```python
from build123d import *

# Parameters (mm, degrees)
SKETCH1_R           = 8.75
BOSS_EXTRUDE1_DEPTH = 13
CUT_EXTRUDE1_REACH  = 19.948
SKETCH2_R           = 2.5
SKETCH3_R           = 4.05
CUT_EXTRUDE2_DEPTH  = 3
CHAMFER1_SIZE       = 0.5


with BuildPart() as part:
    # Sketch1 → Boss-Extrude1 (new body)
    with BuildSketch(Plane(origin=(0, 0, 0), x_dir=(1, 0, 0), z_dir=(0, 1, 0))):
        with Locations(Location((0, 0, 0), (0, 0, 90))):
            Circle(SKETCH1_R)
    extrude(amount=BOSS_EXTRUDE1_DEPTH)

    # Sketch2 → Cut-Extrude1 (cut, up to next)
    with BuildSketch(Plane(origin=(0, 13, 0), x_dir=(1, 0, 0), z_dir=(0, 1, 0)), mode=Mode.PRIVATE) as cut_extrude1_sk1:
        with Locations(Location((0, 0, 0), (0, 0, 270))):
            Circle(SKETCH2_R)
    cut_extrude1_tool1 = extrude(cut_extrude1_sk1.sketch, amount=-CUT_EXTRUDE1_REACH, mode=Mode.PRIVATE) & part.part
    add(cut_extrude1_tool1.solids().sort_by_distance((0, 13, 0))[0], mode=Mode.SUBTRACT)

    # Sketch3 → Cut-Extrude2 (cut)
    with BuildSketch(Plane(origin=(0, 13, 0), x_dir=(1, 0, 0), z_dir=(0, 1, 0))):
        with Locations(Location((0, 0, 0), (0, 0, 270))):
            Circle(SKETCH3_R)
    cut_extrude2 = extrude(amount=-CUT_EXTRUDE2_DEPTH, mode=Mode.SUBTRACT)

    # Mirror3: Cut-Extrude2 across plane
    add(cut_extrude2.mirror(Plane.ZX.offset(6.5)), mode=Mode.SUBTRACT)

    # Chamfer1
    chamfer1_edges = [part.edges().sort_by_distance(p)[0] for p in [
        (0, 13, -4.05),
        (0, 0, -4.05),
    ]]
    chamfer(chamfer1_edges, length=CHAMFER1_SIZE)


solid = part.part
```
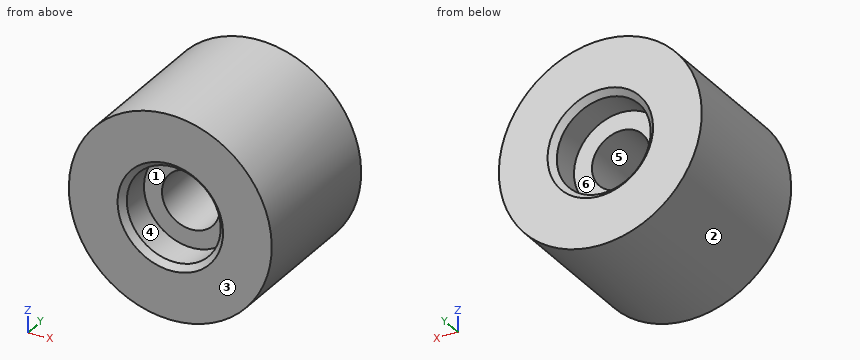
Check sheet for the modelled part. Datum: model origin and axes. Units: mm. Face numbers are marked on the shaded views. A direction names the side the tool comes from. Give positions to 0.01 mm unless a question says otherwise; leave off trailing zeros. Write each loop counter-clockwise with the first axis right and the second up, starting at its lowest first coordinate (ties: lowest second). Pieces come first, ordered by that corner, then holes.
Item 1: Cross-section at D-D (y = 8.5). Enter the section's corners in (x, z).
Item 2: Cross-section at A-A (z = 0). Enter the section's corners in (x, y).
Item 3: Scan lines: L1, parallel to X at y = 2.1, z = 0; L2, parallel to X at y = 7.75, z = 0; L3, parallel to Y at x = 2.75, z = -0.5. Record each from-to range of solid material in increasing order.
Item 4: Cross-section at B-B (x = 0). Enter the section's corners in (y, z).
Item 5: Draft check along X on the marked faces 1, 2 and 3. Enter one of: released by +X, released by -X, zero draft, split by the parting line, or undercut.
Item 6: Gauge pin test, flat ends, axial feed: pin 1 (3 mm diameter, centred on x = 0, z = 0, fed in from -Y); pin 2 (2 mm diameter, centred on x = -4, y = 11, fed in from -Z); pin 3 (6.5 mm diameter, centred on x = 0, z = 0, fed in from -Y); pin 4 (4 mm diameter, centred on y = 11.5, z = -3.5, fed in from -X). Record the tip position at first contact, or that the pin passes through.
Item 7: Cross-section at C-C (y = 2). Enter the section's corners in (x, z), and give its area (3 significant figures).
Item 8: Access from +Z, -Z, +X, -X, +Y, -Y to the whole of each face (thin tool, end or side, straight path). Record for the marked faces 4, 5 and 6.
Report:
1. outline: circle Ø17.5 at (0, 0); hole circle Ø5 at (0, 0)
2. outline: (-8.75, 0) - (-4.55, 0) - (-4.05, 0.5) - (-4.05, 3) - (-2.5, 3) - (-2.5, 10) - (-4.05, 10) - (-4.05, 12.5) - (-4.55, 13) - (-8.75, 13) - close; (2.5, 3) - (4.05, 3) - (4.05, 0.5) - (4.55, 0) - (8.75, 0) - (8.75, 13) - (4.55, 13) - (4.05, 12.5) - (4.05, 10) - (2.5, 10) - close
3. L1: x = -8.75 to -4.05, 4.05 to 8.75
3. L2: x = -8.75 to -2.5, 2.5 to 8.75
3. L3: y = 3 to 10
4. outline: (0, -8.75) - (13, -8.75) - (13, -4.55) - (12.5, -4.05) - (10, -4.05) - (10, -2.5) - (3, -2.5) - (3, -4.05) - (0.5, -4.05) - (0, -4.55) - close; (0, 4.55) - (0.5, 4.05) - (3, 4.05) - (3, 2.5) - (10, 2.5) - (10, 4.05) - (12.5, 4.05) - (13, 4.55) - (13, 8.75) - (0, 8.75) - close
5. face 1: undercut
5. face 2: split by the parting line
5. face 3: zero draft
6. pin 1: passes through
6. pin 2: stops at z = -8.22
6. pin 3: stops at y = 3
6. pin 4: stops at x = -8.62
7. outline: circle Ø17.5 at (0, 0); hole circle Ø8.1 at (0, 0)
7. area: 189 mm2
8. face 4: -Y
8. face 5: +Y, -Y
8. face 6: +Y
